Input: part model. Units: mm. Frame: model coordinates. Face numbers are marked on the shaded views. A direction names the side the tool comes from. Give positions to 0.01 mm unless a question says otherwise; leave off trailing zeros. Loops run counter-clockwise (first coordinate to the right, second up) from the corner with the lowest first, then second, coordinate; pieces in that order, holes last. Notation, with made-up numbers: (-6.5, -10) -> (45.5, -10) arc R22 cw to (45.5, 21) -> close; hole circle Ø8 at (-37, 73.5). An arc over 180 degrees is marked (long way). Answer as a JSON object with one key per item and string values. Group by question number.
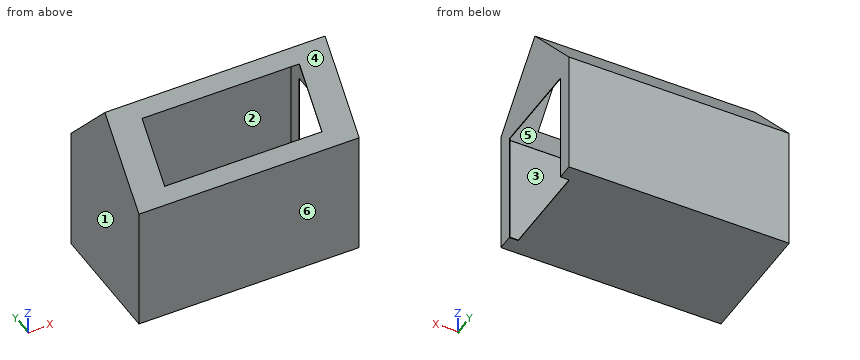
```python
from build123d import *

# Parameters (mm, degrees)
F0_W         = 1066.8
F0_H         = 609.6
F1_DEPTH     = 609.6
F2_T         = -2.54
F3_W         = 457.2
F3_H         = 548.64
F4_DEPTH     = 43.18
F6_DEPTH     = 1066.8
F7_T         = 2.54
F7_T3_DEPTH  = 7.62
F7_T5_DEPTH  = 7.62
F7_T7_DEPTH  = 612.14
F7_T9_DEPTH  = 78.74
F7_T11_DEPTH = 78.74
F7_T13_DEPTH = 1066.8
F7_T15_DEPTH = 609.6
F8_W         = 762
F8_H         = 304.8
F9_DEPTH     = 25.4


# Not quite as in the source:
# - a shell that OpenCascade refuses in one call is made with other operations: the cavity is built on its own and cut out


with BuildPart() as f1:
    # F0 (on Front) → F1 (new body)
    with BuildSketch(Plane.XZ):
        with Locations((533.4, -304.8)):
            Rectangle(F0_W, F0_H)
    extrude(amount=F1_DEPTH)

    # F2
    f2_openings = [f1.faces().sort_by_distance(p)[0] for p in [
        (533.4, -304.8, 0),
    ]]
    offset(amount=F2_T, openings=f2_openings)

    # F3 (on face) → F4 (cut)
    with BuildSketch(Plane.YZ.offset(1066.8)):
        with Locations((-304.8, -335.28)):
            Rectangle(F3_W, F3_H)
    extrude(amount=-F4_DEPTH, mode=Mode.SUBTRACT)

    # F5 (on face) → F6 (join)
    with BuildSketch(Plane(origin=(0, 0, 0), x_dir=(0, -1, 0), z_dir=(-1, 0, 0))):
        Polygon((304.8, 340.776759771), (0, 0), (609.6, 0), align=None)
    extrude(amount=-F6_DEPTH)

    # F7: shell of thickness 2.54, made by hand


with BuildPart() as f7_core1:
    # F7_t2: copy of F1
    add(f1.part)

    # the walls: a layer under each face that stays
    f7_faces = [f7_core1.faces().sort_by_distance(p)[0] for p in [
        (0, -304.8, -134.4116201145),
        (533.4, -304.8, -609.6),
        (533.4, 0, -304.8),
        (533.4, -609.6, -304.8),
        (533.4, -152.4, 170.3883798855),
        (533.4, -457.2, 170.3883798855),
        (1066.8, -304.8, 182.3806331425),
        (1065.3606666667, -76.2, -591.312),
        (1023.62, -304.8, -608.33),
        (1065.3606666667, -533.4, -79.248),
        (1065.53, -304.8, -60.96),
        (1064.26, -563.88, -563.6985714286),
        (533.4, -304.8, -607.06),
        (533.4, -607.06, -303.53),
        (533.4, -2.54, -303.53),
        (2.54, -304.8, -303.53),
    ]]
    thicken(f7_faces, amount=-F7_T, mode=Mode.SUBTRACT)

    # F7_s4 → F7_t3 (cut)
    with BuildSketch(Plane.YZ.offset(1061.72)):
        Polygon((-76.2254, -60.9854), (-73.66, -60.96), (-73.66, -58.42), (-76.2, -58.42), align=None)
        Polygon((-533.3746, -60.9854), (-535.94, -60.96), (-535.94, -58.42), (-533.4, -58.42), align=None)
    extrude(amount=F7_T3_DEPTH, mode=Mode.SUBTRACT)

    # F7_s6 → F7_t5 (cut)
    with BuildSketch(Plane.XY.offset(-612.14)):
        Polygon((1023.6454, -76.2254), (1023.62, -73.66), (1021.08, -73.66), (1021.08, -76.2), align=None)
        Polygon((1023.6454, -533.3746), (1021.08, -533.4), (1021.08, -535.94), (1023.62, -535.94), align=None)
    extrude(amount=F7_T5_DEPTH, mode=Mode.SUBTRACT)

    # F7_s8 → F7_t7 (cut)
    with BuildSketch(Plane.XY.offset(-609.6)):
        Polygon((1064.2346, -607.0346), (1066.8, -607.06), (1066.8, -609.6), (1064.26, -609.6), align=None)
        Polygon((1064.2346, -2.5654), (1066.8, -2.54), (1066.8, 0), (1064.26, 0), align=None)
        Polygon((2.5654, -607.0346), (2.54, -609.6), (0, -609.6), (0, -607.06), align=None)
        Polygon((2.5654, -2.5654), (2.54, 0), (0, 0), (0, -2.54), align=None)
    extrude(amount=F7_T7_DEPTH, mode=Mode.SUBTRACT)

    # F7_s10 → F7_t9 (cut)
    with BuildSketch(Plane.XZ.offset(530.86)):
        Polygon((1064.2346, -607.0346), (1066.8, -607.06), (1066.8, -609.6), (1064.26, -609.6), align=None)
    extrude(amount=F7_T9_DEPTH, mode=Mode.SUBTRACT)

    # F7_s12 → F7_t11 (cut)
    with BuildSketch(Plane.XZ):
        Polygon((1064.2346, -607.0346), (1066.8, -607.06), (1066.8, -609.6), (1064.26, -609.6), align=None)
    extrude(amount=F7_T11_DEPTH, mode=Mode.SUBTRACT)

    # F7_s14 → F7_t13 (cut)
    with BuildSketch(Plane.YZ):
        Polygon((-607.0346, -607.0346), (-607.06, -609.6), (-609.6, -609.6), (-609.6, -607.06), align=None)
        Polygon((-2.5654, -607.0346), (-2.54, -609.6), (0, -609.6), (0, -607.06), align=None)
    extrude(amount=F7_T13_DEPTH, mode=Mode.SUBTRACT)

    # F7_s16 → F7_t15 (cut)
    with BuildSketch(Plane.XZ):
        Polygon((2.5654, -607.0346), (2.54, -609.6), (0, -609.6), (0, -607.06), align=None)
    extrude(amount=F7_T15_DEPTH, mode=Mode.SUBTRACT)


with BuildPart() as f1_1:
    add(f1.part)

    # what is left inside the walls is the cavity
    f7_cavity = [f7_core1.part.solids().sort_by_distance(p)[0] for p in [
        (710.353333, -304.8, 0.0254),
    ]]
    add(f7_cavity, mode=Mode.SUBTRACT)

    # F8 (on face) → F9 (cut)
    with BuildSketch(Plane(origin=(0, -338.6666666667, 302.912675352), x_dir=(1, 0, 0), z_dir=(0, -0.7453559925, 0.6666666667))):
        with Locations((533.4, -177.8)):
            Rectangle(F8_W, F8_H)
    extrude(amount=-F9_DEPTH, mode=Mode.SUBTRACT)


solid = f1_1.part
```
Q1. Pull-direction query (Y, two-part tool) for the marked faces 1, 2, 3 and 4; classes: +Y half, -Y half, draft (parallel to the pull), parting line (faces both ways), or undercut.
Q2. Section A-A on x = 130. Return the cut outline in (y, z).
Q3. Section B-B on y = -388.5. Return the cut outline in (x, z).
Q4. Pin query (flat end, axial travel): pin 1 Ø1.3 at (y, z) = (-368, -608.5) entering from +X; pin 2 Ø1.5 at (y, z) = (-391, -219) entering from +X; pin 3 Ø0.8 at (x, y) = (1066, -348) entering from -Z. Return the tip coordinate at first contact, or that it passes through.
Q5. Section D-D on y = -61.5. Return the cut outline in (x, z).
Q6. Section C-C on z = -269.5. Return the cut outline in (x, y).
Q7. Set-up query: the marked faces 5 and 6. Return all of +Z, -Z, +X, -X, +Y, -Y with unobstructed straight access to the full face (end or side cutting, diameter ignored); none if empty.
Q8. Ray query, probe 1 along X at (y, z) = (-533.5, -28); probe 2 along Y at (x, z) = (694.5, -81); probe 3 along Z at (x, y) = (238, -522.5). Return the intervals inside material, ascending.
Numbers:
{
 "1": {"face 1": "draft", "face 2": "undercut", "face 3": "undercut", "face 4": "-Y half"},
 "2": {"outline": "(-609.6, -609.6) -> (0, -609.6) -> (0, 0) -> (-304.8, 340.78) -> (-609.6, 0) -> close; hole (-607.06, -607.06) -> (-2.54, -607.06) -> (-2.54, 0) -> (-3.41, 0) -> (-304.8, 336.97) -> (-606.19, 0) -> (-607.06, 0) -> close"},
 "3": {"outline": "(0, -609.6) -> (1023.62, -609.6) -> (1023.62, -607.06) -> (2.54, -607.06) -> (2.54, 243.39) -> (152.4, 243.39) -> (152.4, 247.2) -> (0, 247.2) -> close; (914.4, 243.39) -> (1064.26, 243.39) -> (1064.26, -60.96) -> (1066.8, -60.96) -> (1066.8, 247.2) -> (914.4, 247.2) -> close"},
 "4": {"pin 1": "stops at x = 1023.62", "pin 2": "stops at x = 2.54", "pin 3": "stops at z = -60.96"},
 "5": {"outline": "(0, -609.6) -> (1066.8, -609.6) -> (1066.8, 68.76) -> (0, 68.76) -> close; hole (2.54, -607.06) -> (1064.26, -607.06) -> (1064.26, 64.95) -> (2.54, 64.95) -> close"},
 "6": {"outline": "(0, -609.6) -> (1066.8, -609.6) -> (1066.8, -533.4) -> (1064.26, -533.4) -> (1064.26, -607.06) -> (2.54, -607.06) -> (2.54, -2.54) -> (1064.26, -2.54) -> (1064.26, -76.2) -> (1066.8, -76.2) -> (1066.8, 0) -> (0, 0) -> close"},
 "7": {"face 5": "none", "face 6": "+Z, -Z, +X, -X, -Y"},
 "8": {"probe 1": "x = 0 to 2.54, 1064.26 to 1066.8", "probe 2": "y = -609.6 to -607.06, -2.54 to 0", "probe 3": "z = -609.6 to -607.06"}
}
